The model under review builds one solid part; all positions refer to its coordinate system, in mm. Coordinates: 2 decimals unless noted, no trailing zeros. Loops run counter-clockwise (first coordinate to the right, second up) from the corner with the lowest first, then second, coordinate; pieces in that order, holes last. Notation, with made-up numbers: (68.5, 66.25) - (126.5, 66.25) arc R20 ccw to (126.5, 90.25) - close; hole circle Ø9 at (71, 20). An arc over 180 degrees is marked (long way). Answer in a Markdown table with one row per item. Add a question column.
(1) We need section C-C on y = 51.5. Write out the cut boundary in (x, z), plus the area to 3 significant figures.
(2) For P1, Ø10, axis at x = -173, y = 14.5, coming from the -Z side; P2, Ø1.5, axis at y = 67.5, z = 2.5, coming from the -X side, all flat-tipped, find the tip position at first contact; note any pin that passes through.
(3) For line 1 along Y through (x, z) = (-55, 2.2); line 2 along X through (y, z) = (80.5, 2.4); line 3 along X through (y, z) = (131.5, 1.2), list the stretches that pass through material, from the lowest coordinate up.
(4) We need section A-A on z = 2.05. Write out the cut boundary in (x, y), plus the area to 3 significant figures.
(5) We need section B-B on x = -100. Write out the cut boundary in (y, z), plus the area to 3 significant figures.
from build123d import *

# Parameters (mm, degrees)
PAD015_DEPTH                        = 3
SKETCH054_R                         = 1.7
POCKET018_DEPTH                     = 0.001
POCKET018_DEPTH_BACK                = 3.001
BODY001003005003004_PLACEMENT_ANGLE = 60


with BuildPart() as part:
    # Sketch053 → Pad015 (new body)
    with BuildSketch(Plane.XY):
        with BuildLine():
            Line((0, 181.875477), (0, 196.875477))
            ThreePointArc((141.573324, 136.809895), (76.894213, 181.238057), (0, 196.875477))
            ThreePointArc((141.545448, 135.39235), (141.85403, 136.095329), (141.573324, 136.809895))
            Line((132.151008, 126.406294), (141.545448, 135.39235))
            ThreePointArc((130.740934, 126.433766), (131.440303, 126.129123), (132.151008, 126.406294))
            ThreePointArc((130.740934, 126.433766), (71.005238, 167.442364), (0, 181.875477))
        make_face()
    pad015 = extrude(amount=PAD015_DEPTH)

    # Mirrored020: Pad015 across Sketch053 V_Axis
    add(pad015.mirror(Plane(origin=(0, 0, 0), x_dir=(0, 0, 1), z_dir=(1, 0, 0))))

    # Sketch054 → Pocket018 (cut, two sides)
    with BuildSketch(Plane.XY) as pocket018_sk:
        with Locations((129.747586, 137.940691)):
            Circle(SKETCH054_R)
        with Locations((0, 189.372834)):
            Circle(SKETCH054_R)
        with Locations((-129.747586, 137.940691)):
            Circle(SKETCH054_R)
    extrude(amount=-POCKET018_DEPTH, mode=Mode.SUBTRACT)
    extrude(pocket018_sk.sketch, amount=POCKET018_DEPTH_BACK, mode=Mode.SUBTRACT)


with BuildPart() as part_1:
    # Body001003005003004 placement: moved
    add(part.part.rotate(Axis((0, 0, 0), (0, 0, 1)), BODY001003005003004_PLACEMENT_ANGLE))


solid = part_1.part
Outcome:
| question | item | result |
|---|---|---|
| 1 | outline | (-190.02, 0) - (-174.43, 0) - (-174.43, 3) - (-190.02, 3) - close |
| 1 | area | 46.8 mm² |
| 2 | P1 | through |
| 2 | P2 | x = -185.21 |
| 3 | line 1 | 173.36 to 179.69, 182.98 to 189.04 |
| 3 | line 2 | -179.67 to -163.09 |
| 3 | line 3 | -146.52 to -125.64 |
| 4 | outline | (-189.27, -54.2) arc R1 ccw to (-188.03, -54.89) - (-175.55, -51.24) arc R1 ccw to (-174.87, -50.01) arc R181.88 cw to (-44.12, 176.44) arc R1 ccw to (-43.4, 177.65) - (-46.48, 190.28) arc R1 ccw to (-47.69, 191.01) arc R196.88 ccw to (-170.5, 98.44) arc R196.88 ccw to start; hole circle Ø3.4 at (-184.33, -43.39); hole circle Ø3.4 at (-164, 94.69); hole circle Ø3.4 at (-54.59, 181.34) |
| 4 | area | 4,560 mm² |
| 5 | outline | (151.92, 0) - (169.59, 0) - (169.59, 3) - (151.92, 3) - close |
| 5 | area | 53.0 mm² |
